from build123d import *

# Parameters (mm, degrees)
F0_R     = 41.275
F2_R     = 53.594
F5_R     = 3.175
F7_DEPTH = 44.958
F8_DEPTH = 31.75
F9_DEPTH = 6.35
F10_R    = 1.5875


with BuildPart() as f3:
    # F0 (on Top) → F3 section 0
    with BuildSketch(Plane.XY):
        Circle(F0_R)
    # F2 (on offset) → F3 section 1
    with BuildSketch(Plane.XY.offset(83.058)):
        Circle(F2_R)
    loft()

    # F5
    f5_edges = [f3.edges().sort_by_distance(p)[0] for p in [
        (-41.275, 0, 0),
    ]]
    fillet(f5_edges, radius=F5_R)

    # F7 (cut, through all): a face of the model
    f7_faces = [f3.faces().sort_by_distance(p)[0] for p in [
        (0, 0, 83.058),
    ]]
    extrude(f7_faces, amount=-F7_DEPTH, mode=Mode.SUBTRACT)

    # F6 (on offset) → F8 (cut)
    with BuildSketch(Plane.XY.offset(38.1)):
        with BuildLine():
            Line((-24.13, -15.113), (0, -15.113))
            Line((0, -15.113), (0, 15.113))
            Line((0, 15.113), (-10.795, 15.113))
            Line((-10.795, 15.113), (-24.13, 15.113))
            ThreePointArc((-24.13, 15.113), (-26.3750640303, 14.1830640303), (-27.305, 11.938))
            Line((-27.305, 11.938), (-27.305, -11.938))
            ThreePointArc((-27.305, -11.938), (-26.3750640303, -14.1830640303), (-24.13, -15.113))
        make_face()
        with BuildLine():
            Line((0, -15.113), (24.13, -15.113))
            ThreePointArc((24.13, -15.113), (26.3750640303, -14.1830640303), (27.305, -11.938))
            Line((27.305, -11.938), (27.305, 11.938))
            ThreePointArc((27.305, 11.938), (26.3750640303, 14.1830640303), (24.13, 15.113))
            Line((24.13, 15.113), (10.795, 15.113))
            Line((10.795, 15.113), (0, 15.113))
            Line((0, 15.113), (0, -15.113))
        make_face()
    extrude(amount=-F8_DEPTH, mode=Mode.SUBTRACT)

    # F6 (on offset) → F9 (cut)
    with BuildSketch(Plane.XY.offset(38.1)):
        with BuildLine():
            Line((0, -15.113), (24.13, -15.113))
            ThreePointArc((24.13, -15.113), (26.3750640303, -14.1830640303), (27.305, -11.938))
            Line((27.305, -11.938), (27.305, 11.938))
            ThreePointArc((27.305, 11.938), (26.3750640303, 14.1830640303), (24.13, 15.113))
            Line((24.13, 15.113), (10.795, 15.113))
            Line((10.795, 15.113), (0, 15.113))
            Line((0, 15.113), (0, -15.113))
        make_face()
        with BuildLine():
            Line((-24.13, -15.113), (0, -15.113))
            Line((0, -15.113), (0, 15.113))
            Line((0, 15.113), (-10.795, 15.113))
            Line((-10.795, 15.113), (-24.13, 15.113))
            ThreePointArc((-24.13, 15.113), (-26.3750640303, 14.1830640303), (-27.305, 11.938))
            Line((-27.305, 11.938), (-27.305, -11.938))
            ThreePointArc((-27.305, -11.938), (-26.3750640303, -14.1830640303), (-24.13, -15.113))
        make_face()
        with BuildLine():
            Line((-10.795, 15.113), (0, 15.113))
            Line((0, 15.113), (10.795, 15.113))
            Line((10.795, 15.113), (10.795, 23.6855))
            ThreePointArc((10.795, 23.6855), (10.3300320151, 24.8080320151), (9.2075, 25.273))
            Line((9.2075, 25.273), (-9.2075, 25.273))
            ThreePointArc((-9.2075, 25.273), (-10.3300320151, 24.8080320151), (-10.795, 23.6855))
            Line((-10.795, 23.6855), (-10.795, 15.113))
        make_face()
    extrude(amount=-F9_DEPTH, mode=Mode.SUBTRACT)

    # F10
    f10_edges = [f3.edges().sort_by_distance(p)[0] for p in [
        (0, 15.113, 31.75),
        (0, -15.113, 6.35),
        (26.375064, -14.183064, 6.35),
        (27.305, 0, 6.35),
        (26.375064, 14.183064, 6.35),
        (0, 15.113, 6.35),
        (-26.375064, 14.183064, 6.35),
        (-27.305, 0, 6.35),
        (-26.375064, -14.183064, 6.35),
        (-46.925917, 0, 38.1),
        (0, -15.113, 38.1),
        (26.375064, -14.183064, 38.1),
        (27.305, 0, 38.1),
        (26.375064, 14.183064, 38.1),
        (17.4625, 15.113, 38.1),
        (10.795, 19.39925, 38.1),
        (10.330032, 24.808032, 38.1),
        (0, 25.273, 38.1),
        (-10.330032, 24.808032, 38.1),
        (-10.795, 19.39925, 38.1),
        (-17.4625, 15.113, 38.1),
        (-26.375064, 14.183064, 38.1),
        (-27.305, 0, 38.1),
        (-26.375064, -14.183064, 38.1),
    ]]
    fillet(f10_edges, radius=F10_R)


solid = f3.part
Read the model definition and answer for the solid it produces. Units are mm, in the model's axes. A direction names the side the tool comes from. Coordinates: 2 decimals unless noted, no trailing zeros. Loops run counter-clockwise (first coordinate to the right, second up) from the corner with the lowest first, then second, coordinate; pieces in that order, holes last.
Q1. The mould has two halves that part along X. Classify faces 3 (the face through (-1, 1, 0)), 4 (the face through (0, 25.273, 34)), 5 (the face through (23.167, 36.338, 12.269)), 6 (the face through (-26.4, -14.16, 22.43)): +X half, -X half, draft (parallel to the pull), parting line (faces both ways), or undercut.
Q2. Which of the six approach directions +Z, -Z, +X, -X, +Y, -Y give full straight-line access (tool end or side, diameter ignored) to faces 1 (the face through (27.305, 0, 22)), 2 (the face through (-1, -19, 38.1))?
Q3. Consider probe 1 along Z at (x, y) = (0.5, 7); probe 2 along Y at (x, z) = (-1, 19.5); probe 3 along X at (y, z) = (-8, 17) (3 decimals). Determine where each line is inside the solid, lowest interval first.
Q4. Each of these flat-tipped pins is pushed along its axis until it touches: pin 1 Ø12 at (x, z) = (-21.5, 18.5) entering from +Y; pin 2 Ø2.5 at (x, z) = (0, 34) entering from -Y; pin 3 Ø3 at (y, z) = (20, 32) entering from +X; pin 4 Ø4 at (x, y) = (10, -7.5) entering from -Z. Where does it stop, or does it pass through?
Q5. The part is cut by section C-C on z = 4.5. Write down the section's boundary in (x, y).
Results below:
1. face 3: draft
1. face 4: undercut
1. face 5: parting line
1. face 6: undercut
2. face 1: +Z
2. face 2: +Z, +X, -X, +Y, -Y
3. probe 1: z = 0 to 6.35
3. probe 2: y = -44.16 to -15.11, 15.11 to 44.16
3. probe 3: x = -43.06 to -27.305, 27.305 to 43.06
4. pin 1: stops at y = 41.39
4. pin 2: stops at y = -46.5
4. pin 3: stops at x = 42.18
4. pin 4: stops at z = 0
5. outline: circle Ø83.88 at (0, 0)
